from build123d import *

# Parameters (mm, degrees)
F1_R     = 2.251249
F2_DEPTH = 42.926
F3_DEPTH = 25.4


with BuildPart() as f2:
    # F1 (on Right) → F2 (new body)
    with BuildSketch(Plane.YZ):
        Circle(F1_R)
    extrude(amount=F2_DEPTH)

    # F0 (on Front) → F3 (join)
    with BuildSketch(Plane.XZ):
        Polygon((44.636123, 0), (41.285951, 0), (37.344571, 0), (37.344571, -1.872155), (44.636123, -1.872155), align=None)
        Polygon((37.344571, 0), (41.285951, 0), (44.636123, 0), (44.636123, 1.872155), (37.344571, 1.872155), align=None)
        Polygon((37.344571, 3.356544), (37.344571, 1.872155), (44.636123, 1.872155), (44.661563, 1.872155), (44.661563, 3.356544), align=None)
    extrude(amount=F3_DEPTH)


solid = f2.part
The listing builds one solid part. Answer for the finished solid, in the listing's coordinates (mm). A direction names the side the tool comes from. Round coordinates to 2 decimals unless told otherwise and drop trailing zeros. Order: outer loops, then holes, each group sorted by start corner. A loop starts at its lowest first (then second) coordinate and runs counter-clockwise, first axis right, second up. Notation, with made-up numbers: M -38,56 L 7,56 A18 cw 7,78 Z; hole C -11,-19.5 d4. An arc over 180 degrees is marked long. Answer in a Markdown table with one row per item. Add a question column.
1) Flat-ended cylindrical pins translate along their axes: pin 1 Ø1 at (x, z) = (37.5, 1) entering from +Y (3 decimals); pin 2 Ø1.5 at (x, y) = (38.5, -13) entering from -Z; pin 3 Ø3 at (y, z) = (0, -0.5) entering from +X. Find the tip coordinate at first contact, or state that the pin passes through.
2) Which of the six approach directions +Z, -Z, +X, -X, +Y, -Y give full straight-line access (tool end or side, diameter ignored) to faces 1 (the face through (21.16, 2.08, -0.86)), 2 (the face through (43, 0, 3)), 3 (the face through (41, -13, 3.357))?
3) The part is cut by section A-A on z = 0. Determine the outline of the cut face in (x, y).
4) The part is cut by section C-C on x = 33.5. Determine the outline of the cut face in (y, z).
5) Consider line 1 along X through (y, z) = (-22.75, 2.45); line 2 along X through (y, z) = (-18.25, 0.9); line 3 along Z through (x, y) = (43, -5.25). Determine where each line is inside the solid, lowest interval first. Write a range as from..to.
Findings below:
| question | item | result |
|---|---|---|
| 1 | pin 1 | stops at y = 2.195 |
| 1 | pin 2 | stops at z = -1.87 |
| 1 | pin 3 | stops at x = 44.64 |
| 2 | face 1 | -X |
| 2 | face 2 | +Z, +X, +Y |
| 2 | face 3 | +Z, +X, -X, +Y, -Y |
| 3 | outline | M 0,-2.25 L 37.34,-2.25 L 37.34,-25.4 L 44.64,-25.4 L 44.64,0 L 42.93,0 L 42.93,2.25 L 0,2.25 Z |
| 4 | outline | C 0,0 d4.5 |
| 5 | line 1 | x = 37.34..44.66 |
| 5 | line 2 | x = 37.34..44.64 |
| 5 | line 3 | z = -1.87..3.36 |
